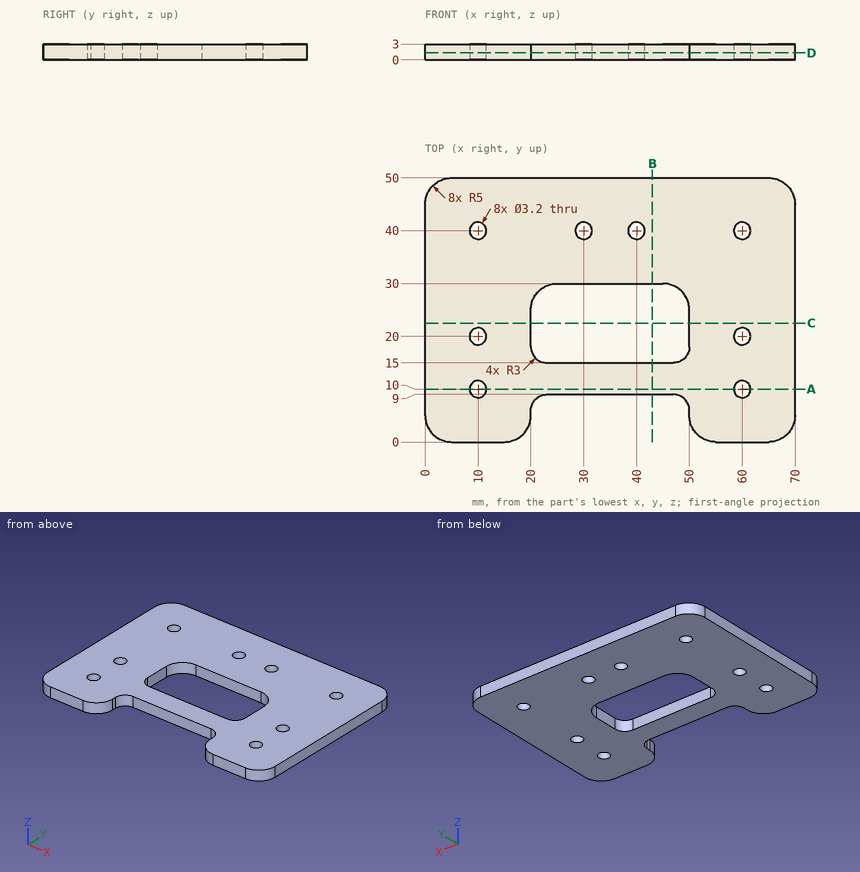
Input: dimensioned drawing with shaded views. Units: mm. Origin: part minimum x, y, z. Coordinates: 2 decimals unless noted, no trailing zeros. Loops run counter-clockwise (first coordinate to the right, second up) from the corner with the lowest first, then second, coordinate; pieces in that order, holes last. Notation, with made-up numbers: (53, 45.25) -> (86, 45.25) arc R10 cw to (86, 56.25) -> close; hole circle Ø4 at (86, 57.5). An arc over 180 degrees is marked (long way). Use a Markdown table: item, result. Add a question column.
(1) Pin query (flat end, axial travel): pin 1 Ø1 at (x, y) = (20.5, 28.5) entering from -Z; pin 2 Ø0.9 at (x, z) = (36, 1.5) entering from -Y; pin 3 Ø1 at (x, z) = (51, 2) entering from -Y. Return the tip coordinate at first contact, or that it passes through.
(2) Section query A-A, the plane y = 10. Return loops of the section in (x, z), plus the area to 3 significant figures.
(3) Line query: line 1 along Y through (x, z) = (40, 0.95); line 2 along Y through (x, z) = (10, 0.8); line 3 along Y through (x, z) = (28, 2.2). Output: solid intervals per line, ascending.
(4) Section query D-D, the plane z = 1.3. State how many separate pieces and enclosed holes the cut face has, plus the area to 3 significant figures.
(5) Section query B-B, the plane x = 43. Return loops of the section in (y, z).
(6) Section query C-C, the plane y = 22.5. Return loops of the section in (x, z), plus the area to 3 significant figures.
Answer:
| question | item | result |
|---|---|---|
| 1 | pin 1 | stops at z = 0 |
| 1 | pin 2 | stops at y = 9 |
| 1 | pin 3 | stops at y = 1.43 |
| 2 | outline | (0, 0) -> (8.4, 0) -> (8.4, 3) -> (0, 3) -> close; (11.6, 0) -> (58.4, 0) -> (58.4, 3) -> (11.6, 3) -> close; (61.6, 0) -> (70, 0) -> (70, 3) -> (61.6, 3) -> close |
| 2 | area | 191 mm^2 |
| 3 | line 1 | y = 9 to 15, 30 to 38.4, 41.6 to 50 |
| 3 | line 2 | y = 0 to 8.4, 11.6 to 18.4, 21.6 to 38.4, 41.6 to 50 |
| 3 | line 3 | y = 9 to 15, 30 to 50 |
| 4 | separate pieces | 1 |
| 4 | enclosed holes | 9 |
| 4 | area | 2,700 mm^2 |
| 5 | outline | (9, 0) -> (15, 0) -> (15, 3) -> (9, 3) -> close; (30, 0) -> (50, 0) -> (50, 3) -> (30, 3) -> close |
| 6 | outline | (0, 0) -> (20, 0) -> (20, 3) -> (0, 3) -> close; (50, 0) -> (70, 0) -> (70, 3) -> (50, 3) -> close |
| 6 | area | 120 mm^2 |
